Here's the drawing with two shaded views (mm, measured from the low corner). I have some questions. A direction names the side the tool comes from. Round coordinates to 2 decimals unless told otherwise and drop trailing zeros. Loops run counter-clockwise (first coordinate to the right, second up) from the corner with the lowest first, then second, coordinate; pieces in that order, holes last.
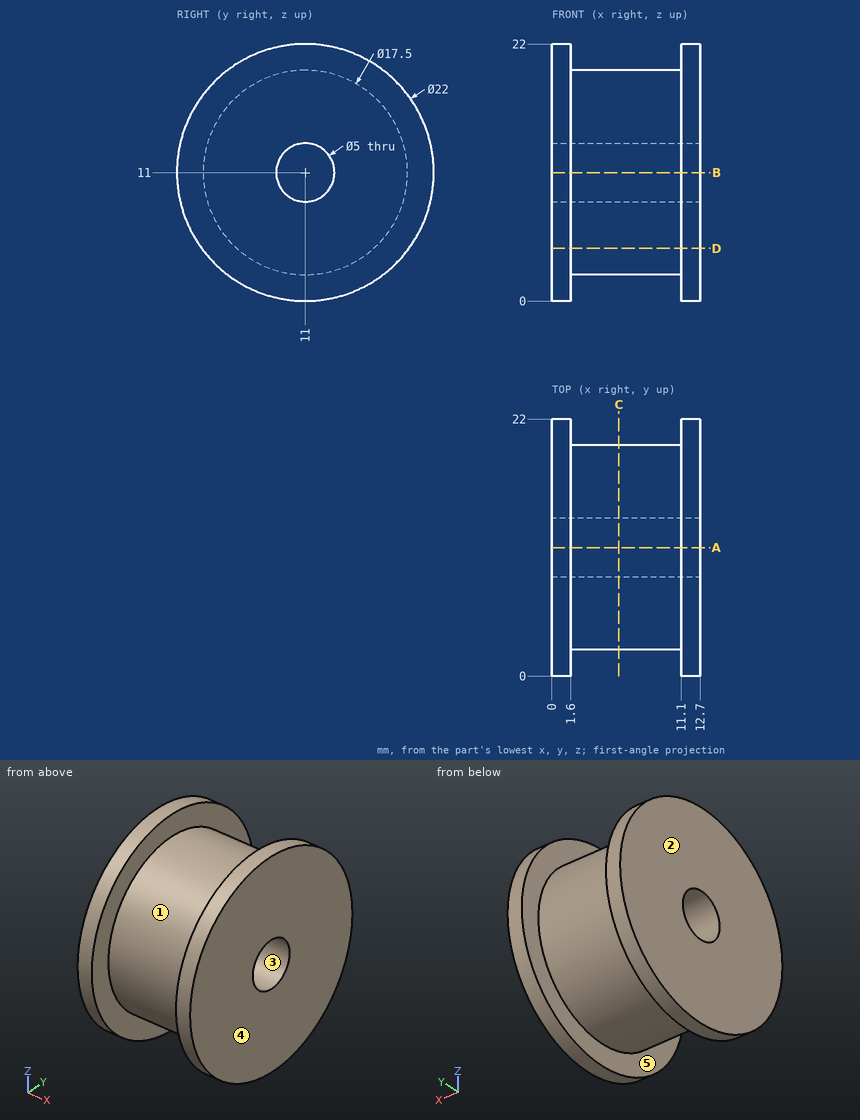
Item 1: For the marked faces 4 and 5, which set-ups out of +Z, -Z, +X, -X, +Y, -Y let a thin tool reach every point of the face, with its end or its side?
Results list:
face 4: +Z, -Z, +X, +Y, -Y
face 5: none
Item 2: If we section it at D-D, the plane z = 4.5: Please give me the cut outline in (x, y).
Results list:
outline: (0, 2.13) - (1.6, 2.13) - (1.6, 5.14) - (11.1, 5.14) - (11.1, 2.13) - (12.7, 2.13) - (12.7, 19.87) - (11.1, 19.87) - (11.1, 16.86) - (1.6, 16.86) - (1.6, 19.87) - (0, 19.87) - close
Item 3: We'd pull the mould along Y, two halves only. Please class the marked faces 1, 2 and 3: released by +Y, released by -Y, zero draft, split by the parting line, or undercut.
Results list:
face 1: split by the parting line
face 2: zero draft
face 3: undercut
Item 4: If we section it at C-C, the plane x = 5.75: Please give me the cut outline in (y, z), then the cut area to 3 significant figures.
Results list:
outline: circle Ø17.5 at (11, 11); hole circle Ø5 at (11, 11)
area: 221 mm2
Item 5: If we section it at A-A, the plane y = 11: Please give me the cut outline in (x, z), then the cut area to 3 significant figures.
Results list:
outline: (0, 0) - (1.6, 0) - (1.6, 2.25) - (11.1, 2.25) - (11.1, 0) - (12.7, 0) - (12.7, 8.5) - (0, 8.5) - close; (0, 13.5) - (12.7, 13.5) - (12.7, 22) - (11.1, 22) - (11.1, 19.75) - (1.6, 19.75) - (1.6, 22) - (0, 22) - close
area: 173 mm2
Item 6: If I drill on line 1 along Z through (x, y) = (4.75, 11); line 2 along X through (y, z) = (9.75, 1.25); line 3 along Z through (x, y) = (5.5, 11.5), over which ranges is the centre line in solid material (lowest first)?
Results list:
line 1: z = 2.25 to 8.5, 13.5 to 19.75
line 2: x = 0 to 1.6, 11.1 to 12.7
line 3: z = 2.26 to 8.55, 13.45 to 19.74
Item 7: Will these pins go through, and if not, where does the flat tip stop? pin 1 (6 mm diameter, centred on x = 7.5, y = 2.5, fed in from -Z); pin 2 (3 mm diameter, centred on x = 11, z = 4, fed in from -Y); pin 3 (1 mm diameter, centred on x = 7.5, z = 11, fed in from -Y).
Results list:
pin 1: stops at z = 4.19
pin 2: stops at y = 1.48
pin 3: stops at y = 2.25
